Autodesk Inventor part; units mm, degrees
ref_plane "YZ Plane" through (0, 0, 0) normal (1, 0, 0) x (0, 1, 0)
ref_plane "XZ Plane" through (0, 0, 0) normal (0, 1, 0) x (-1, 0, 0)
ref_plane "XY Plane" through (0, 0, 0) normal (0, 0, 1) x (1, 0, 0)
sketch "Szkic1" plane through (0, 0, 0) normal (0, 1, 0) x (-1, 0, 0)
  line L0 (8.4728, 9.9771) -> (-0.5272, 9.9771)
  line L1 (-0.5272, 9.9771) -> (-0.5272, -10.0229)
  line L2 (-0.5272, -10.0229) -> (8.4728, -10.0229)
  line L3 (8.4728, -10.0229) -> (8.4728, 9.9771)
  point P0 (0, 0)
  dimension "d0" = 9
  dimension "d1" = 20
extrude "Wyciągnięcie proste1" add sketch "Szkic1" along normal blind 1.6
fillet "Zaokrąglenie1" radius 0.6 4 edges at (-8.4728, 0.8, -10.0229) (0.5272, 0.8, -10.0229) (0.5272, 0.8, 9.9771) (-8.4728, 0.8, 9.9771)
sketch "Szkic2" plane through (0, 0, 0) normal (0, -1, 0) x (1, 0, 0)
  circle A0 centre (-1.9728, -6.1673) radius 0.75
  circle A1 centre (-1.9728, -6.1673) radius 1.25
  point P0 (0, 0)
  dimension "d5" = 2.5
extrude "Wyciągnięcie proste2" cut sketch "Szkic2" against normal through all contours A0 | A1
sketch "Szkic4" plane through (0, 1.6, 0) normal (0, 1, 0) x (1, 0, 0)
  line L0 (-0.0728, 10.0229) -> (-7.8728, 10.0229)
  circle A0 centre (-1.9728, 6.1673) radius 1.25
  line L1 (-3.9728, 10.0229) -> (-3.9728, -9.9771)
  line L2 (-7.8728, -9.9771) -> (-0.0728, -9.9771)
  circle A1 centre (-5.9728, 6.1673) radius 1.25
  point P0 (0, 0)
extrude "Wyciągnięcie proste3" cut sketch "Szkic4" against normal blind 10 contours A1
sketch "Szkic5" plane through (0, 1.6, 0) normal (0, 1, 0) x (1, 0, 0)
  circle A0 centre (-5.9728, 6.1673) radius 1.25
  circle A1 centre (-1.9728, 6.1673) radius 1.25
  arc A2 (-8.4728, -9.3771) -> (-7.8728, -9.9771) centre (-7.8728, -9.3771) ccw
  line L0 (-7.8728, -9.9771) -> (-0.0728, -9.9771)
  arc A3 (-0.0728, -9.9771) -> (0.5272, -9.3771) centre (-0.0728, -9.3771) ccw
  line L1 (0.5272, -9.3771) -> (0.5272, 9.4229)
  arc A4 (0.5272, 9.4229) -> (-0.0728, 10.0229) centre (-0.0728, 9.4229) ccw
  line L2 (-0.0728, 10.0229) -> (-7.8728, 10.0229)
  arc A5 (-7.8728, 10.0229) -> (-8.4728, 9.4229) centre (-7.8728, 9.4229) ccw
  line L3 (-8.4728, 9.4229) -> (-8.4728, -9.3771)
  point P0 (0, 0)
properties part number "pcb_czujnik"
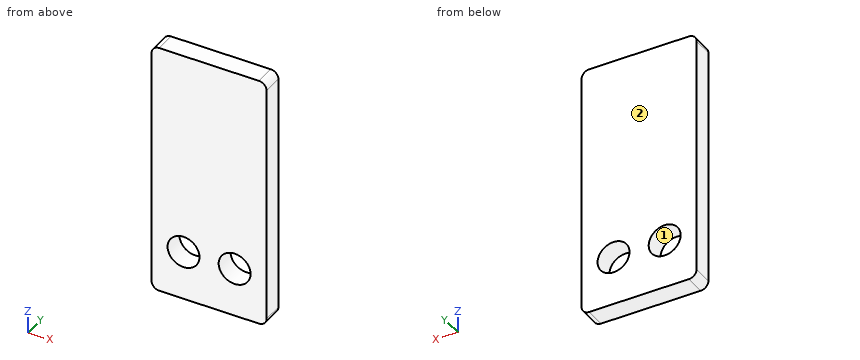
Geometry check sheet. Reference: the model listing, model coordinates, mm. Face numbers are marked on the shaded views. Coordinates: 2 decimals unless noted, no trailing zeros. Order: outer loops, then holes, each group sorted by start corner. A loop starts at its lowest first (then second) coordinate and runs counter-clockwise, first axis right, second up.
Item 1: Section check D-D (x = -7). Enter the section's corners in (y, z) (3 decimals), plus the area to 3 significant figures.
Item 2: Depth check by flat-ended pin: pin 1 (3 mm diameter, centred on x = -3, z = 6.5, fed in from -Y). Enter the tip coordinate at first touch or a pass-through.
Item 3: Section check A-A (x = -5). Enter the section's corners in (y, z).
Item 4: Scan lines: line 1 along Z through (x, y) = (-6.75, 1.4); line 2 along X through (y, z) = (1.15, -6.5); line 3 along Z through (x, y) = (0, 1). Record each from-to range of solid material in increasing order.
Item 5: Section check B-B (z = -6.5). Enter the section's corners in (x, y), plus the area to 3 significant figures.
Item 6: Section check C-C (y = 1.15). Enter the section's corners in (x, z), plus the area to 3 significant figures.
Item 7: Mould release check, pull along Z, two halves, no side actions. Record for the marked faces 1 and 2: released by +Z, released by -Z, zero draft, split by the parting line, or undercut.
Check sheet entries:
1. outline: (0, -10.023) - (1.6, -10.023) - (1.6, -6.88) - (0, -6.88) - close; (0, -5.455) - (1.6, -5.455) - (1.6, 9.977) - (0, 9.977) - close
1. area: 29.7 mm2
2. pin 1: stops at y = 0
3. outline: (0, -10.02) - (1.6, -10.02) - (1.6, -6.95) - (0, -6.95) - close; (0, -5.38) - (1.6, -5.38) - (1.6, 9.98) - (0, 9.98) - close
4. line 1: z = -10.02 to -7.15, -5.19 to 9.98
4. line 2: x = -8.47 to -7.18, -4.77 to -3.18, -0.77 to 0.53
4. line 3: z = -10.02 to 9.97
5. outline: (-8.47, 0) - (-7.18, 0) - (-7.18, 1.6) - (-8.47, 1.6) - close; (-4.77, 0) - (-3.18, 0) - (-3.18, 1.6) - (-4.77, 1.6) - close; (-0.77, 0) - (0.53, 0) - (0.53, 1.6) - (-0.77, 1.6) - close
5. area: 6.69 mm2
6. outline: (-8.47, -9.42) arc R0.6 ccw to (-7.87, -10.02) - (-0.07, -10.02) arc R0.6 ccw to (0.53, -9.42) - (0.53, 9.38) arc R0.6 ccw to (-0.07, 9.98) - (-7.87, 9.98) arc R0.6 ccw to (-8.47, 9.38) - close; hole circle Ø2.5 at (-5.97, -6.17); hole circle Ø2.5 at (-1.97, -6.17)
6. area: 170 mm2
7. face 1: undercut
7. face 2: zero draft
